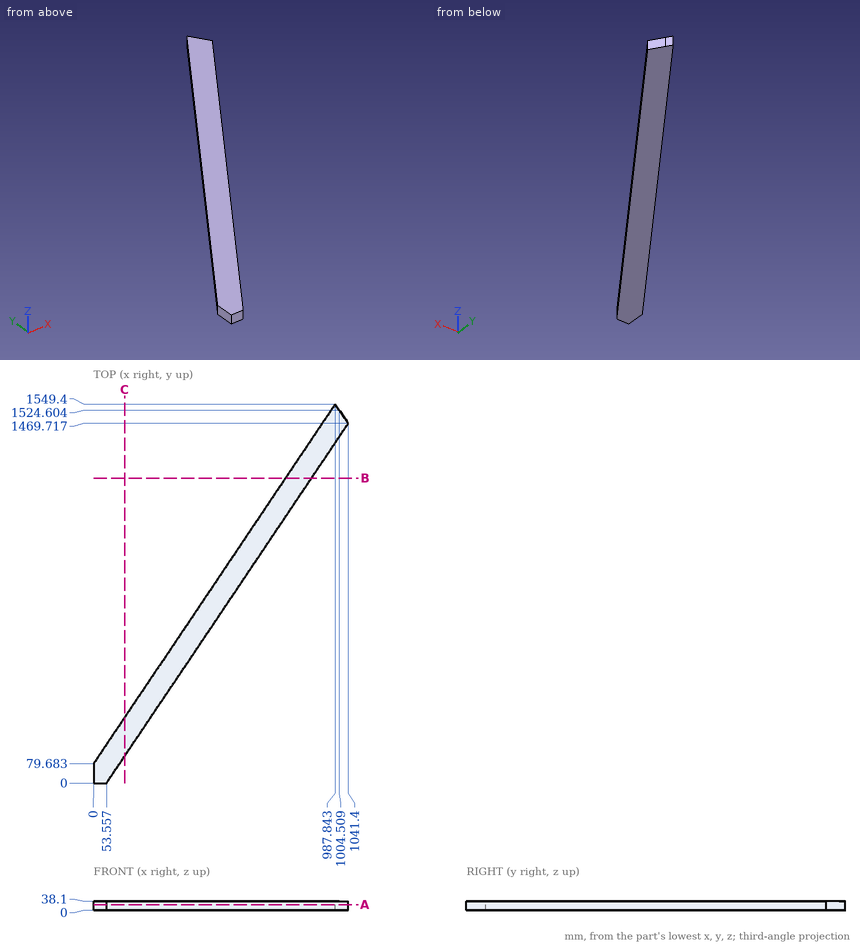
Drawing for the job (mm, zero at the part's lowest x, y, z). Round coordinates to 2 decimals unless told otherwise and drop trailing zeros. Loops run counter-clockwise (first coordinate to the right, second up) from the corner with the lowest first, then second, coordinate; pieces in that order, holes last. Notation, with made-up numbers: M -2.5,8 L 27.5,8 A35 ccw 27.5,40 Z; hole C -9,77.5 d8. An arc over 180 degrees is marked long. Use a Markdown table: item, result. Add a question column.
(1) Flat gauge pins, fed straight in: pin 1 (5 mm diameter, centred on y = 980, z = 25.5, fed in from +X); pin 2 (1 mm diameter, centred on x = 216, z = 29.5, fed in from -Y); pin 3 (12 mm diameter, centred on y = 654, z = 34, fed in from -X). Where does each tip first touch, or does it go through?
(2) Cut at C-C (x = 127.5). Give the cut face in (y, z).
(3) Drill centre lines: line 1 (X direction, y = 243, z = 10.5) (1 decimal); line 2 (X direction, y = 637, z = 33) (1 decimal); line 3 (Y direction, x = 198.5, z = 3.5) (1 decimal). Where is each one in solid material? Low to high.
(4) Cut at B-B (y = 1246). Give the cut face in (x, z), and give its area (3 significant figures).
(5) Cut at A-A (z = 24). Give the cut face in (x, y).
Geometry says:
| question | item | result |
|---|---|---|
| 1 | pin 1 | stops at x = 713.93 |
| 1 | pin 2 | stops at y = 240.94 |
| 1 | pin 3 | stops at x = 381.98 |
| 2 | outline | M 110.01,0 L 269.38,0 L 269.38,38.1 L 110.01,38.1 Z |
| 3 | line 1 | x = 109.8 to 216.9 |
| 3 | line 2 | x = 374.6 to 481.7 |
| 3 | line 3 | y = 215.6 to 375 |
| 4 | outline | M 783.92,0 L 891.03,0 L 891.03,38.1 L 783.92,38.1 Z |
| 4 | area | 4,080 mm² |
| 5 | outline | M 0,0 L 53.56,0 L 1041.4,1469.72 L 1004.51,1524.6 L 987.84,1549.4 L 0,79.68 Z |
